Geometry: final body of the model. Coordinates: model frame, mm. A direction names the side the tool comes from. Coordinates: 2 decimals unless noted, no trailing zeros. Write each loop counter-clockwise with the first axis right and the second up, starting at its lowest first coordinate (ties: lowest second). Pieces come first, ordered by that corner, then holes. Notation, with made-up numbers: (-8, -5.5) - (6, -5.5) arc R24 cw to (6, 20.5) - close; hole circle Ø1 at (9, 87). An arc over 180 degrees is marked (long way). Answer as a JSON object with one key per item and string values. Group by question number.
Item 1: Line query: line 1 along Z through (x, y) = (-60, 3.7); line 2 along X through (y, z) = (1.45, 25); line 3 along X through (y, z) = (3.6, 25). Output: solid intervals per line, ascending. Write a range as from..to.
Item 2: Section C-C on x = -29.5. Return loops of the section in (y, z).
Item 3: Section B-B on z = 19.5. Return loops of the section in (x, y).
Item 4: Set-up query: faces 1 (the flat face through (-1, 1, 0)), 2 (the flat face through (-24.7, 0.5, 31)), 3 (the cylindrical face through (27.9, 0.51, 21.86)). Return all of +Z, -Z, +X, -X, +Y, -Y with unobstructed straight access to the full face (end or side cutting, diameter ignored); none if empty.
Item 5: Section A-A on y = 2.2. Return loops of the section in (x, z).
Item 6: Mould query, pull axis Z, two halves, no side actions, for faces 4 (the cylindrical face through (56.1, 0.51, 21.86)), 5 (the flat face through (-0.3, 0.8, -31)), 6 (the cylindrical face through (-60.29, 3.7, 26.32)). Classes: pulls with the +Z half, pulls with the -Z half, needs draft (parallel to the pull), parting line crosses it, or undercut.
Item 7: First-contact query: pin 1 Ø12 at (x, z) = (32.5, 2.5) entering from +Y; pin 2 Ø1.1 at (x, y) = (46, 0.5) entering from +Z; pin 3 Ø0.6 at (x, z) = (58, -24.5) entering from -Y. Flat tips, straight axial feed; report the tip coordinate or a pass-through.
```python
from build123d import *

# Parameters (mm, degrees)
SKETCH1_W           = 126
SKETCH1_H           = 62
BOSS_EXTRUDE1_DEPTH = 1
SKETCH2_W           = 6
SKETCH2_H           = 62
BOSS_EXTRUDE2_DEPTH = 3
SKETCH3_R           = 1.35
CUT_EXTRUDE1_DEPTH  = 5
SKETCH4_R           = 2.5
CUT_EXTRUDE2_DEPTH  = 3
SKETCH5_W           = 30
SKETCH5_H           = 10
CUT_EXTRUDE3_DEPTH  = 5
FILLET1_R           = 3
CUT_EXTRUDE4_DEPTH  = 0.2
SKETCH7_W           = 2.7
SKETCH7_H           = 2.7
CUT_EXTRUDE5_DEPTH  = 0.2
SKETCH8_W           = 0.3
SKETCH8_H           = 62
CUT_EXTRUDE6_DEPTH  = 5


with BuildPart() as part:
    # Sketch1 → Boss-Extrude1 (new body)
    with BuildSketch(Plane(origin=(0, 0, 0), x_dir=(1, 0, 0), z_dir=(0, 1, 0))):
        Rectangle(SKETCH1_W, SKETCH1_H)
    extrude(amount=BOSS_EXTRUDE1_DEPTH)

    # Sketch2 → Boss-Extrude2 (add)
    with BuildSketch(Plane(origin=(0, 1, 0), x_dir=(1, 0, 0), z_dir=(0, 1, 0))):
        with Locations((-60, 0)):
            Rectangle(SKETCH2_W, SKETCH2_H)
        with Locations((60, 0)):
            Rectangle(SKETCH2_W, SKETCH2_H)
    extrude(amount=BOSS_EXTRUDE2_DEPTH)

    # Sketch3 → Cut-Extrude1 (cut, through all)
    with BuildSketch(Plane(origin=(0, 4, 0), x_dir=(1, 0, 0), z_dir=(0, 1, 0))):
        with Locations((-60, 25)):
            Circle(SKETCH3_R)
        with Locations((-60, -25)):
            Circle(SKETCH3_R)
        with Locations((60, -25)):
            Circle(SKETCH3_R)
        with Locations((60, 25)):
            Circle(SKETCH3_R)
    extrude(amount=-CUT_EXTRUDE1_DEPTH, mode=Mode.SUBTRACT)

    # Sketch4 → Cut-Extrude2 (cut)
    with BuildSketch(Plane.XZ):
        with Locations((60, -25)):
            Circle(SKETCH4_R)
        with Locations((60, 25)):
            Circle(SKETCH4_R)
        with Locations((-60, 25)):
            Circle(SKETCH4_R)
        with Locations((-60, -25)):
            Circle(SKETCH4_R)
    extrude(amount=-CUT_EXTRUDE2_DEPTH, mode=Mode.SUBTRACT)

    # Sketch5 → Cut-Extrude3 (cut, through all)
    with BuildSketch(Plane.XZ):
        with Locations((42, 26)):
            Rectangle(SKETCH5_W, SKETCH5_H)
    extrude(amount=-CUT_EXTRUDE3_DEPTH, mode=Mode.SUBTRACT)

    # Fillet1
    fillet1_edges = [part.edges().sort_by_distance(p)[0] for p in [
        (27, 0.5, 21),
        (57, 0.5, 21),
    ]]
    fillet(fillet1_edges, radius=FILLET1_R)

    # Sketch6 → Cut-Extrude4 (cut)
    with BuildSketch(Plane.XZ.offset(-3)):
        with BuildLine():
            Line((-61.35, 22.895837459), (-61.35, 27.104162541))
            ThreePointArc((-61.35, 27.104162541), (-60, 27.5), (-58.65, 27.104162541))
            Line((-58.65, 27.104162541), (-58.65, 22.895837459))
            ThreePointArc((-58.65, 22.895837459), (-60, 22.5), (-61.35, 22.895837459))
        make_face()
        with BuildLine():
            Line((-61.35, -27.104162541), (-61.35, -22.895837459))
            ThreePointArc((-61.35, -22.895837459), (-60, -22.5), (-58.65, -22.895837459))
            Line((-58.65, -22.895837459), (-58.65, -27.104162541))
            ThreePointArc((-58.65, -27.104162541), (-60, -27.5), (-61.35, -27.104162541))
        make_face()
    cut_extrude4 = extrude(amount=-CUT_EXTRUDE4_DEPTH, mode=Mode.SUBTRACT)

    # Sketch7 → Cut-Extrude5 (cut)
    with BuildSketch(Plane.XZ.offset(-3.2)):
        with Locations((-60, -25)):
            Rectangle(SKETCH7_W, SKETCH7_H)
        with Locations((-60, 25)):
            Rectangle(SKETCH7_W, SKETCH7_H)
    cut_extrude5 = extrude(amount=-CUT_EXTRUDE5_DEPTH, mode=Mode.SUBTRACT)

    # Mirror1: Cut-Extrude4, Cut-Extrude5 across plane
    add(cut_extrude4.mirror(Plane(origin=(0, 0, 0), x_dir=(0, 0, 1), z_dir=(1, 0, 0))), mode=Mode.SUBTRACT)
    add(cut_extrude5.mirror(Plane(origin=(0, 0, 0), x_dir=(0, 0, 1), z_dir=(1, 0, 0))), mode=Mode.SUBTRACT)

    # Sketch8 → Cut-Extrude6 (cut, through all)
    with BuildSketch(Plane(origin=(0, 4, 0), x_dir=(1, 0, 0), z_dir=(0, 1, 0))):
        with Locations((-62.85, 0)):
            Rectangle(SKETCH8_W, SKETCH8_H)
        with Locations((62.85, 0)):
            Rectangle(SKETCH8_W, SKETCH8_H)
    extrude(amount=-CUT_EXTRUDE6_DEPTH, mode=Mode.SUBTRACT)


solid = part.part
```
Checks:
{
 "1": {"line 1": "-31..-26.35, -23.65..23.65, 26.35..31", "line 2": "-62.7..-62.5, -57.5..-57, 57..57.5, 62.5..62.7", "line 3": "-62.7..-61.35, -58.65..-57, 57..58.65, 61.35..62.7"},
 "2": {"outline": "(0, -31) - (1, -31) - (1, 31) - (0, 31) - close"},
 "3": {"outline": "(-62.7, 0) - (62.7, 0) - (62.7, 4) - (57, 4) - (57, 1) - (-57, 1) - (-57, 4) - (-62.7, 4) - close"},
 "4": {"face 1": "+Z, -Z, +Y", "face 2": "+Z, +X, -X, +Y, -Y", "face 3": "+Z, +Y, -Y"},
 "5": {"outline": "(-62.7, -31) - (-57, -31) - (-57, 31) - (-62.7, 31) - close; (57, -31) - (62.7, -31) - (62.7, 31) - (57, 31) - close; hole circle Ø5 at (-60, -25); hole circle Ø5 at (-60, 25); hole circle Ø5 at (60, -25); hole circle Ø5 at (60, 25)"},
 "6": {"face 4": "pulls with the +Z half", "face 5": "pulls with the -Z half", "face 6": "undercut"},
 "7": {"pin 1": "y = 1", "pin 2": "z = 21", "pin 3": "y = 3"}
}
